The listing builds one solid part. Answer for the finished solid, in the listing's coordinates (mm). Coordinates: 2 decimals unless noted, no trailing zeros. Write each loop counter-clockwise with the first axis right and the second up, starting at its lowest first coordinate (ties: lowest second). Pieces come first, ordered by that corner, then holes.
from build123d import *

# Parameters (mm, degrees)
SKETCH1_RX         = 60.325
SKETCH1_RY         = 44.45
BASE_EXTRUDE_DEPTH = 3.175


with BuildPart() as part:
    # Sketch1 → Base-Extrude (new body)
    with BuildSketch(Plane.XY):
        with BuildLine():
            Line((-752.475, -70.773505599), (-701.7766, -339.075622164))
            ThreePointArc((-701.7766, -339.075622164), (0.530014677, -273.05003733), (702.818, -339.273481384))
            Line((702.818, -339.273481384), (752.475, -70.773505599))
            ThreePointArc((752.475, -70.773505599), (0, 0), (-752.475, -70.773505599))
        make_face()
        with Locations(Location((-527.440710052, -182.216417238), (0, 0, -93.81))):
            Ellipse(SKETCH1_RX, SKETCH1_RY, mode=Mode.SUBTRACT)
    extrude(amount=-BASE_EXTRUDE_DEPTH)


solid = part.part
Q1. The part is cut by section A-A, the plane x = -326. Write down the section's boundary in (y, z) (3 decimals).
Answers below:
outline: (-287.199, -3.175) - (-13.189, -3.175) - (-13.189, 0) - (-287.199, 0) - close
Q2. Given pin 1 (1 mm diameter, centred on x = -574.5, z = -1.5, fed in from +Y), flat-ended and moving along its own axis, determine where the tip first touches the part or whether it passes through.
Answers below:
pin 1: stops at y = -41.03
Q3. The part is cut by section B-B, the plane x = 593.5. Write down the section's boundary in (y, z) (3 decimals), then the cut area to 3 significant figures.
Answers below:
outline: (-320.154, -3.175) - (-43.88, -3.175) - (-43.88, 0) - (-320.154, 0) - close
area: 877 mm2
Q4. Find the intervals of material crossed by probe 1 along X at (y, z) = (-71, -0.35); probe 2 along X at (y, z) = (-160.5, -1.3); probe 3 along Y at (x, z) = (-11.5, -2.6), in increasing order.
Answers below:
probe 1: x = -752.43 to 752.43
probe 2: x = -735.52 to -568.29, -485.28 to 735.88
probe 3: y = -273.07 to -0.02
Q5. Determine the mould class of faces 1 (the face through (-9.36, -273.06, -1.57)), 2 (the face through (-11, -167, -3.175)), 3 (the face through (727.3, -206.9, -1.6)), 4 (the face through (-727.48, -203.05, -1.57)) for opening direction X: released by +X, released by -X, zero draft, split by the parting line, or undercut.
Answers below:
face 1: undercut
face 2: zero draft
face 3: released by +X
face 4: released by -X
